Design review of the part built by this model. Coordinates are the model's own, in mm. A direction names the side the tool comes from. Coordinates: 2 decimals unless noted, no trailing zeros. Order: outer loops, then holes, each group sorted by start corner. A loop starts at its lowest first (then second) coordinate and runs counter-clockwise, first axis right, second up. Notation, with made-up numbers: M 42,52.5 L 55,52.5 A18 cw 55,56.5 Z; hole C -7,38.25 d4. An arc over 180 degrees is marked long. Answer as a JSON object with one key per item and string values.
from build123d import *

# Parameters (mm, degrees)
BOSS_EXTRUDE1_DEPTH = 6.2
BOSS_EXTRUDE2_DEPTH = 21
CHAMFER1_SIZE       = 5
CHAMFER1_SIZE2      = 28.356409098
CUT_EXTRUDE1_REACH  = 74.109
CHAMFER2_SIZE       = 1
CHAMFER2_SIZE2      = 9.514364454
CHAMFER3_SIZE       = 2
CUT_EXTRUDE2_REACH  = 79.092
CUT_EXTRUDE3_START  = -3.468867
CUT_EXTRUDE3_DEPTH  = 3.468867
BOSS_EXTRUDE3_DEPTH = 6.2
CUT_EXTRUDE4_REACH  = 79.092


with BuildPart() as part:
    # Sketch1 → Boss-Extrude1 (new body)
    with BuildSketch(Plane.XY):
        with BuildLine():
            Line((-28.3, 0), (0, 0))
            Line((0, 0), (0, 10))
            Line((0, 10), (-7.1, 10))
            ThreePointArc((-7.1, 10), (-14.171067812, 12.928932188), (-17.1, 20))
            Line((-17.1, 20), (-17.1, 51))
            Line((-17.1, 51), (-20.1, 51))
            Line((-20.1, 51), (-20.1, 6))
            Line((-20.1, 6), (-24.3, 6))
            Line((-24.3, 6), (-24.3, 50))
            Line((-24.3, 50), (-28.3, 50))
            Line((-28.3, 50), (-28.3, 0))
        make_face()
    extrude(amount=BOSS_EXTRUDE1_DEPTH)

    # Sketch2 → Boss-Extrude2 (add)
    with BuildSketch(Plane.XZ):
        Polygon((0, 6.2), (0, 10.4), (11, 10.4), (11, 42.4), (-24.1, 42.4), (-24.1, 10.4), (-13.1, 10.4), (-13.1, 6.2), align=None)
    extrude(amount=-BOSS_EXTRUDE2_DEPTH)

    # Chamfer1
    chamfer1_edges = [part.edges().sort_by_distance(p)[0] for p in [
        (-6.55, 0, 42.4),
    ]]
    chamfer1_side = [part.faces().sort_by_distance(p)[0] for p in [
        (-6.55, 10.5, 42.4),
    ]]
    chamfer(chamfer1_edges, length=CHAMFER1_SIZE, length2=CHAMFER1_SIZE2, reference=chamfer1_side[0])

    # Sketch3 → Cut-Extrude1 (cut, up to next)
    with BuildSketch(Plane(origin=(0, 0, 0), x_dir=(0, 0, -1), z_dir=(1, 0, 0)), mode=Mode.PRIVATE) as cut_extrude1_sk1:
        Polygon((-6.2, 10), (-7.6, 10), (-10.4, 21), (-6.2, 21), align=None)
    cut_extrude1_tool1 = extrude(cut_extrude1_sk1.sketch, amount=-CUT_EXTRUDE1_REACH, mode=Mode.PRIVATE) & part.part
    add(cut_extrude1_tool1.solids().sort_by_distance((0, 16.416667, 7.716667))[0], mode=Mode.SUBTRACT)

    # Chamfer2
    chamfer2_edges = [part.edges().sort_by_distance(p)[0] for p in [
        (11, 10.5, 10.4),
    ]]
    chamfer2_side = [part.faces().sort_by_distance(p)[0] for p in [
        (11, 11.541747932, 25.62778603),
    ]]
    chamfer(chamfer2_edges, length=CHAMFER2_SIZE, length2=CHAMFER2_SIZE2, reference=chamfer2_side[0])

    # Chamfer3
    chamfer3_edges = [part.edges().sort_by_distance(p)[0] for p in [
        (-24.1, 10.5, 10.4),
    ]]
    chamfer(chamfer3_edges, length=CHAMFER3_SIZE)

    # Sketch5 → Cut-Extrude2 (cut, up to next)
    with BuildSketch(Plane(origin=(11, 0, 0), x_dir=(0, 0, -1), z_dir=(1, 0, 0)), mode=Mode.PRIVATE) as cut_extrude2_sk1:
        Polygon((-42.4, 17.8), (-13.86886709, 5), (-10.966215349, -4.108657177), (-44.036924755, 0.937700744), align=None)
    cut_extrude2_tool1 = extrude(cut_extrude2_sk1.sketch, amount=-CUT_EXTRUDE2_REACH, mode=Mode.PRIVATE) & part.part
    add(cut_extrude2_tool1.solids().sort_by_distance((11, 5.258773, 29.627692))[0], mode=Mode.SUBTRACT)

    # Sketch6 → Cut-Extrude3 (cut)
    with BuildSketch(Plane(origin=(0, 0, 10.4), x_dir=(-1, 0, 0), z_dir=(0, 0, -1)).offset(CUT_EXTRUDE3_START)):
        Polygon((13.1, 0), (24.1, 5), (37.198342989, 5), (28.62602328, -4.522208447), (-13.825974113, -5.629287686), (-20.705007466, 5), (-11, 5), (0, 0), align=None)
    extrude(amount=CUT_EXTRUDE3_DEPTH, mode=Mode.SUBTRACT)

    # Sketch7 → Boss-Extrude3 (add)
    with BuildSketch(Plane.XY.offset(6.2)):
        with BuildLine():
            Line((-16.7, 50.6), (-15.7, 50.5))
            ThreePointArc((-15.7, 50.5), (-15.462165524, 50.365875857), (-15.4, 50.1))
            ThreePointArc((-15.4, 50.1), (-15.462165524, 49.834124143), (-15.7, 49.7))
            Line((-15.7, 49.7), (-16.7, 49.6))
            ThreePointArc((-16.7, 49.6), (-16.971392676, 49.471392676), (-17.1, 49.2))
            Line((-17.1, 49.2), (-17.1, 48.7))
            ThreePointArc((-17.1, 48.7), (-16.971392676, 48.428607324), (-16.7, 48.3))
            Line((-16.7, 48.3), (-15.7, 48.2))
            ThreePointArc((-15.7, 48.2), (-15.462165524, 48.065875857), (-15.4, 47.8))
            ThreePointArc((-15.4, 47.8), (-15.462165524, 47.534124143), (-15.7, 47.4))
            Line((-15.7, 47.4), (-16.7, 47.3))
            ThreePointArc((-16.7, 47.3), (-16.971392676, 47.171392676), (-17.1, 46.9))
            Line((-17.1, 46.9), (-17.1, 46.4))
            ThreePointArc((-17.1, 46.4), (-16.971392676, 46.128607324), (-16.7, 46))
            Line((-16.7, 46), (-15.7, 45.9))
            ThreePointArc((-15.7, 45.9), (-15.462165524, 45.765875857), (-15.4, 45.5))
            ThreePointArc((-15.4, 45.5), (-15.462165524, 45.234124143), (-15.7, 45.1))
            Line((-15.7, 45.1), (-16.7, 45))
            ThreePointArc((-16.7, 45), (-16.971392676, 44.871392676), (-17.1, 44.6))
            Line((-17.1, 44.6), (-17.1, 44.1))
            ThreePointArc((-17.1, 44.1), (-16.971392676, 43.828607324), (-16.7, 43.7))
            Line((-16.7, 43.7), (-15.7, 43.6))
            ThreePointArc((-15.7, 43.6), (-15.462165524, 43.465875857), (-15.4, 43.2))
            ThreePointArc((-15.4, 43.2), (-15.462165524, 42.934124143), (-15.7, 42.8))
            Line((-15.7, 42.8), (-16.7, 42.7))
            ThreePointArc((-16.7, 42.7), (-16.971392676, 42.571392676), (-17.1, 42.3))
            Line((-17.1, 42.3), (-17.1, 41.8))
            ThreePointArc((-17.1, 41.8), (-16.971392676, 41.528607324), (-16.7, 41.4))
            Line((-16.7, 41.4), (-15.7, 41.3))
            ThreePointArc((-15.7, 41.3), (-15.462165524, 41.165875857), (-15.4, 40.9))
            ThreePointArc((-15.4, 40.9), (-15.462165524, 40.634124143), (-15.7, 40.5))
            Line((-15.7, 40.5), (-16.7, 40.4))
            ThreePointArc((-16.7, 40.4), (-16.971392676, 40.271392676), (-17.1, 40))
            Line((-17.1, 40), (-17.1, 39.5))
            ThreePointArc((-17.1, 39.5), (-16.971392676, 39.228607324), (-16.7, 39.1))
            Line((-16.7, 39.1), (-15.7, 39))
            ThreePointArc((-15.7, 39), (-15.462165524, 38.865875857), (-15.4, 38.6))
            ThreePointArc((-15.4, 38.6), (-15.462165524, 38.334124143), (-15.7, 38.2))
            Line((-15.7, 38.2), (-16.7, 38.1))
            ThreePointArc((-16.7, 38.1), (-16.971392676, 37.971392676), (-17.1, 37.7))
            Line((-17.1, 37.7), (-17.1, 37.2))
            ThreePointArc((-17.1, 37.2), (-16.971392676, 36.928607324), (-16.7, 36.8))
            Line((-16.7, 36.8), (-15.7, 36.7))
            ThreePointArc((-15.7, 36.7), (-15.462165524, 36.565875857), (-15.4, 36.3))
            ThreePointArc((-15.4, 36.3), (-15.462165524, 36.034124143), (-15.7, 35.9))
            Line((-15.7, 35.9), (-16.7, 35.8))
            ThreePointArc((-16.7, 35.8), (-16.971392676, 35.671392676), (-17.1, 35.4))
            Line((-17.1, 35.4), (-17.1, 34.9))
            ThreePointArc((-17.1, 34.9), (-16.971392676, 34.628607324), (-16.7, 34.5))
            Line((-16.7, 34.5), (-15.7, 34.4))
            ThreePointArc((-15.7, 34.4), (-15.462165524, 34.265875857), (-15.4, 34))
            ThreePointArc((-15.4, 34), (-15.462165524, 33.734124143), (-15.7, 33.6))
            Line((-15.7, 33.6), (-16.7, 33.5))
            ThreePointArc((-16.7, 33.5), (-16.971392676, 33.371392676), (-17.1, 33.1))
            Line((-17.1, 33.1), (-17.1, 32.6))
            ThreePointArc((-17.1, 32.6), (-16.971392676, 32.328607324), (-16.7, 32.2))
            Line((-16.7, 32.2), (-15.7, 32.1))
            ThreePointArc((-15.7, 32.1), (-15.462165524, 31.965875857), (-15.4, 31.7))
            ThreePointArc((-15.4, 31.7), (-15.462165524, 31.434124143), (-15.7, 31.3))
            Line((-15.7, 31.3), (-16.7, 31.2))
            ThreePointArc((-16.7, 31.2), (-16.971392676, 31.071392676), (-17.1, 30.8))
            Line((-17.1, 30.8), (-17.1, 30.3))
            ThreePointArc((-17.1, 30.3), (-16.971392676, 30.028607324), (-16.7, 29.9))
            Line((-16.7, 29.9), (-15.7, 29.8))
            ThreePointArc((-15.7, 29.8), (-15.462165524, 29.665875857), (-15.4, 29.4))
            ThreePointArc((-15.4, 29.4), (-15.462165524, 29.134124143), (-15.7, 29))
            Line((-15.7, 29), (-16.7, 28.9))
            ThreePointArc((-16.7, 28.9), (-16.971392676, 28.771392676), (-17.1, 28.5))
            Line((-17.1, 28.5), (-17.1, 28))
            ThreePointArc((-17.1, 28), (-16.971392676, 27.728607324), (-16.7, 27.6))
            Line((-16.7, 27.6), (-15.7, 27.5))
            ThreePointArc((-15.7, 27.5), (-15.462165524, 27.365875857), (-15.4, 27.1))
            ThreePointArc((-15.4, 27.1), (-15.462165524, 26.834124143), (-15.7, 26.7))
            Line((-15.7, 26.7), (-16.7, 26.6))
            ThreePointArc((-16.7, 26.6), (-16.971392676, 26.471392676), (-17.1, 26.2))
            Line((-17.1, 26.2), (-17.1, 25.7))
            ThreePointArc((-17.1, 25.7), (-16.971392676, 25.428607324), (-16.7, 25.3))
            Line((-16.7, 25.3), (-15.7, 25.2))
            ThreePointArc((-15.7, 25.2), (-15.462165524, 25.065875857), (-15.4, 24.8))
            ThreePointArc((-15.4, 24.8), (-15.462165524, 24.534124143), (-15.7, 24.4))
            Line((-15.7, 24.4), (-16.7, 24.3))
            ThreePointArc((-16.7, 24.3), (-16.971392676, 24.171392676), (-17.1, 23.9))
            Line((-17.1, 23.9), (-17.1, 23.4))
            ThreePointArc((-17.1, 23.4), (-16.971392676, 23.128607324), (-16.7, 23))
            Line((-16.7, 23), (-15.7, 22.9))
            ThreePointArc((-15.7, 22.9), (-15.462165524, 22.765875857), (-15.4, 22.5))
            ThreePointArc((-15.4, 22.5), (-15.462165524, 22.234124143), (-15.7, 22.1))
            Line((-15.7, 22.1), (-16.7, 22))
            ThreePointArc((-16.7, 22), (-16.971392676, 21.871392676), (-17.1, 21.6))
            Line((-17.1, 21.6), (-17.1, 21.1))
            ThreePointArc((-17.1, 21.1), (-16.971392676, 20.828607324), (-16.7, 20.7))
            Line((-16.7, 20.7), (-15.7, 20.6))
            ThreePointArc((-15.7, 20.6), (-15.462165524, 20.465875857), (-15.4, 20.2))
            ThreePointArc((-15.4, 20.2), (-15.462165524, 19.934124143), (-15.7, 19.8))
            Line((-15.7, 19.8), (-16.7, 19.7))
            ThreePointArc((-16.7, 19.7), (-16.971392676, 19.571392676), (-17.1, 19.3))
            Line((-17.1, 19.3), (-17.1, 18.8))
            Line((-17.1, 18.8), (-18.685, 49.2))
            Line((-18.685, 49.2), (-17.1, 51))
            ThreePointArc((-17.1, 51), (-16.971392676, 50.728607324), (-16.7, 50.6))
        make_face()
    extrude(amount=-BOSS_EXTRUDE3_DEPTH)

    # Sketch8 → Cut-Extrude4 (cut, up to next)
    with BuildSketch(Plane(origin=(11, 0, 0), x_dir=(0, 0, -1), z_dir=(1, 0, 0)), mode=Mode.PRIVATE) as cut_extrude4_sk1:
        Polygon((-35.4, 21), (-27.4, 17), (-19.4, 21), align=None)
    cut_extrude4_tool1 = extrude(cut_extrude4_sk1.sketch, amount=-CUT_EXTRUDE4_REACH, mode=Mode.PRIVATE) & part.part
    add(cut_extrude4_tool1.solids().sort_by_distance((11, 19.666667, 27.4))[0], mode=Mode.SUBTRACT)


solid = part.part
1) To check wall thickness, follow L1, parallel to Y at x = -1, z = 11; L2, parallel to Z at x = -24.5, y = 37; L3, parallel to Z at x = 1, y = 19. State the ranges of each line that lie inside material, in increasing order.
Taken from the geometry:
{"L1": "y = 0 to 21", "L2": "z = 0 to 6.2", "L3": "z = 10.4 to 23.4, 31.4 to 42.4"}
2) Mouldability with a two-part tool opening along X and no side actions: class faces 1 (the flat face through (-20.1, 29, 3)), 2 (the flat face through (-13.1, 8, 9)), 3 (the flat face through (-22, 6, 3)), 4 (the flat face through (-26, 50, 3)) as released by +X, released by -X, zero draft, split by the parting line, or undercut.
Taken from the geometry:
{"face 1": "undercut", "face 2": "released by -X", "face 3": "undercut", "face 4": "zero draft"}
3) Add section D-D (z = 32). State the section outline as (x, y) points.
Taken from the geometry:
{"outline": "M -24.1,13.13 L 11,13.13 L 11,19.3 L -24.1,19.3 Z"}
4) Insertion check: pin 1 Ø0.6 at (y, z) = (44.5, 4.5) entering from +X; pin 2 Ø4 at (x, z) = (3, 17) entering from +Y; pin 3 Ø3 at (x, z) = (-3, 16.5) entering from -Y; pin 4 Ø1 at (y, z) = (5.5, 21) entering from -X. Each pin has a flat end and moves straight along its axis. Give the tip position at first contact, or say it passes through.
Taken from the geometry:
{"pin 1": "stops at x = -17.03", "pin 2": "stops at y = 21", "pin 3": "stops at y = 5.51", "pin 4": "passes through"}
5) Tool access review of faces 5 (the flat face through (0, 6, 6)), 6 (the flat face through (-6.304, 11.49, 28.334)), 7 (the flat face through (-18.523, 2.465, 11.773)), 8 (the flat face through (-5, 10, 5)): name each direction out of +Z, -Z, +X, -X, +Y, -Y from which nothing blocks a thin tool from reaching the whole face with its end or side.
Taken from the geometry:
{"face 5": "-Z, +X, +Y, -Y", "face 6": "+Z, +X, -X, -Y", "face 7": "+Z, -X, -Y", "face 8": "+X, +Y"}
6) Add section C-C (x = 5). State the section outline as (y, z) points.
Taken from the geometry:
{"outline": "M 2.27,10.77 L 21,10.77 L 21,19.4 L 17,27.4 L 21,35.4 L 21,42.4 L 17.8,42.4 L 5,13.87 L 2.27,13 Z"}
7) Add section A-A (x = -11). State the section outline as (y, z) points, and give its area (3 significant figures).
Taken from the geometry:
{"outline": "M 0,0 L 10.79,0 L 10.79,6.2 L 10,6.2 L 10,7.6 L 21,10.4 L 21,19.4 L 17,27.4 L 21,35.4 L 21,42.4 L 17.8,42.4 L 5,13.87 L 0,12.28 Z", "area": "435 mm2"}
8) Add section B-B (z = 21). State the section outline as (x, y) points.
Taken from the geometry:
{"outline": "M -24.1,8.2 L 11,8.2 L 11,20.2 L -24.1,20.2 Z"}
